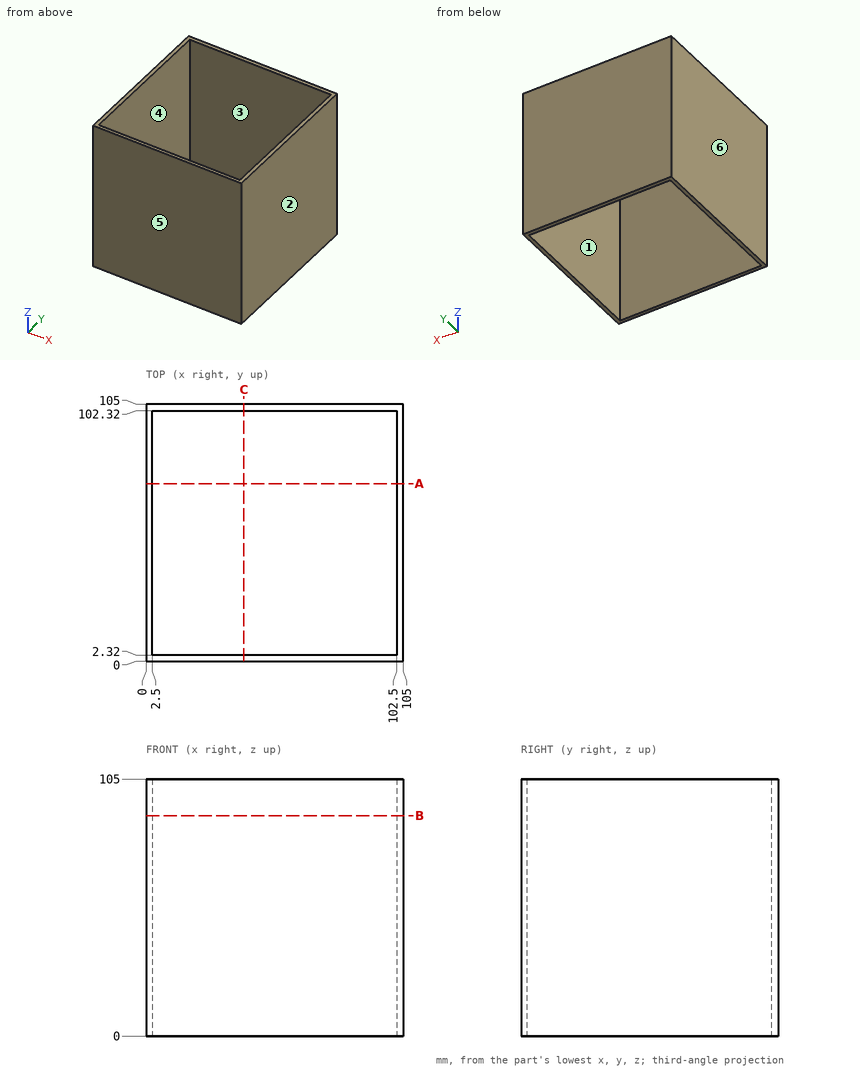
Geometry: see drawing. Coordinates: mm, zero at the bounding-box minimum. A direction names the side the tool comes from. Give positions to 0.01 mm unless a question says otherwise; leave off trailing zeros. Loops run counter-clockwise (first coordinate to the right, second up) from the corner with the lowest first, then second, coordinate; pieces in that order, holes last. Notation, with made-up numbers: (86.25, 38.25) - (145.25, 38.25) arc R32 cw to (145.25, 68.25) - close; hole circle Ø9 at (23, 13.5). An arc over 180 degrees is marked (long way). Answer as CSV lines item,"result". Start each with the question number.
1. Section C-C, the plane x = 40. Return loops of the section in (y, z).
2. Section B-B, the plane z = 90. Return loops of the section in (x, y).
3. Draft query along Y for the marked faces 3, 4, 5 and 6. Return one class per face: released by +Y, released by -Y, zero draft, split by the parting line, or undercut.
4. Reachability of the marked faces 1 and 2 from +Z, -Z, +X, -X, +Y, -Y: full face, straight path, thin tool, end or side. Return the list, or none.
5. Section A-A, the plane y = 72.5. Return loops of the section in (x, z).
6. Ray query, L1, parallel to Y at x = 67.5, z = 19.5; L2, parallel to X at y = 52, z = 86. Return the intervals inside material, ascending.
Answers:
1,outline,"(0, 0) - (2.32, 0) - (2.32, 105) - (0, 105) - close; (102.32, 0) - (105, 0) - (105, 105) - (102.32, 105) - close"
2,outline,"(0, 0) - (105, 0) - (105, 105) - (0, 105) - close; hole (2.5, 2.32) - (102.5, 2.32) - (102.5, 102.32) - (2.5, 102.32) - close"
3,face 3,"undercut"
3,face 4,"undercut"
3,face 5,"released by -Y"
3,face 6,"zero draft"
4,face 1,"+Z, -Z"
4,face 2,"+Z, -Z, +X, +Y, -Y"
5,outline,"(0, 0) - (2.5, 0) - (2.5, 105) - (0, 105) - close; (102.5, 0) - (105, 0) - (105, 105) - (102.5, 105) - close"
6,L1,"y = 0 to 2.32, 102.32 to 105"
6,L2,"x = 0 to 2.5, 102.5 to 105"
